For this review, take the finished solid that the model builds, in its own axes (mm). A direction names the side the tool comes from. Coordinates: 2 decimals unless noted, no trailing zeros. Order: outer loops, then holes, each group sorted by start corner. A loop starts at its lowest first (then second) coordinate and runs counter-clockwise, first axis right, second up.
Autodesk Fusion 360 part; units mm, degrees
sketch "Sketch1" plane through (0, 0, 0) normal (0, 0, 1) x (1, 0, 0)
  line L0 (20, -20) -> (-20, -20)
  line L1 (-20, -20) -> (-20, 20)
  line L2 (-20, 20) -> (20, 20)
  line L3 (20, 20) -> (20, -20)
  line L4 (20, -20) -> (-20, 20) construction
  line L5 (-20, -20) -> (20, 20) construction
  line L6 (12.5, -12.5) -> (-12.5, -12.5) construction
  line L7 (-12.5, -12.5) -> (-12.5, 12.5) construction
  line L8 (-12.5, 12.5) -> (12.5, 12.5) construction
  line L9 (12.5, 12.5) -> (12.5, -12.5) construction
  line L10 (12.5, -12.5) -> (-12.5, 12.5) construction
  line L11 (-12.5, -12.5) -> (12.5, 12.5) construction
  circle A0 centre (-12.5, 12.5) radius 2.25
  circle A1 centre (12.5, 12.5) radius 2.25
  circle A2 centre (12.5, -12.5) radius 2.25
  circle A3 centre (-12.5, -12.5) radius 2.25
  dimension "d1" = 40
  dimension "d2" = 40
  dimension "d3" = 25
  dimension "d4" = 25
  dimension "d5" = 4.5
  dimension "d6" = 4.5
  dimension "d7" = 4.5
  dimension "d8" = 4.5
extrude "Extrude1" add sketch "Sketch1" along normal blind 4
sketch "Sketch2" plane through (0, 0, 4) normal (0, 0, 1) x (-1, 0, 0)
  circle A0 centre (12.5, 12.5) radius 2.25
  circle A1 centre (12.5, -12.5) radius 2.25
  circle A2 centre (-12.5, -12.5) radius 2.25
  circle A3 centre (-12.5, 12.5) radius 2.25
  line L0 (-20, -20) -> (20, -20)
  line L1 (20, -20) -> (20, 20)
  line L2 (20, 20) -> (-20, 20)
  line L3 (-20, 20) -> (-20, -20)
  circle A4 centre (0, 0) radius 10.3
  circle A5 centre (0, 0) radius 12.3
  dimension "d11" = 20.6
  dimension "d12" = 2
extrude "Extrude2" add sketch "Sketch2" along normal blind 30 contours A5
sketch "Sketch3" plane through (0, 0, 0) normal (1, 0, 0) x (0, 1, 0)
  line L0 (12.3, 34) -> (-12.3, 34)
  line L1 (-12.3, 4) -> (12.3, 4)
  line L2 (-12.3, 34) -> (12.3, 4) construction
  circle A0 centre (0, 19) radius 2.1
  dimension "d15" = 4.2
extrude "Extrude3" cut sketch "Sketch3" along normal through all and the other way through all
fillet "Fillet1" radius 2 1 edges at (11.4676, -4.4479, 4)
1. Take a section at C-C, the plane x = 0. Give the boundary of the cut face in (y, z).
Answer below:
outline: (-20, 0) - (20, 0) - (20, 4) - (14.3, 4) arc R2 cw to (12.3, 6) - (12.3, 34) - (10.3, 34) - (10.3, 4) - (-10.3, 4) - (-10.3, 34) - (-12.3, 34) - (-12.3, 6) arc R2 cw to (-14.3, 4) - (-20, 4) - close
2. Clearance check with flat-ended pins moving along their axes: pin 1 Ø6 at (x, y) = (-12.5, 12.5) entering from -Z; pin 2 Ø6 at (x, y) = (-4, 3.5) entering from +Z; pin 3 Ø8 at (x, z) = (4, 10) entering from -Y; pin 4 Ø6.5 at (y, z) = (0, 19) entering from +X. State where each tip first meets the part, or that it passes through.
Answer below:
pin 1: stops at z = 0
pin 2: stops at z = 4
pin 3: stops at y = -12.3
pin 4: stops at x = 12.3
3. Take a section at B-B, the plane z = 13.5. Give the boundary of the cut face in (x, y), plus the area to 3 significant figures.
Answer below:
outline: circle Ø24.6 at (0, 0); hole circle Ø20.6 at (0, 0)
area: 142 mm2
4. To check wall thickness, follow L1, parallel to Y at x = 12.5, z = 0.8; L2, parallel to Z at x = 11.25, y = 0; L3, parallel to X at y = -12, z = 2. State the ranges of each line that lie inside material, in increasing order.
Answer below:
L1: y = -20 to -14.75, -10.25 to 10.25, 14.75 to 20
L2: z = 0 to 16.9, 21.1 to 34
L3: x = -20 to -14.69, -10.31 to 10.31, 14.69 to 20
5. Take a section at D-D, the plane x = -11.5. Give the number of separate pieces and of enclosed holes in the cut face, plus the area to 3 significant figures.
Answer below:
separate pieces: 3
enclosed holes: 1
area: 380 mm2
6. The part is to be moulded in two halves that separate along Y. For faces 1 (the face through (-5.4, 9.1, 34)), 2 (the face through (0, -20, 2)), 3 (the face through (-14.16, -14.02, 1.97)), 4 (the face through (11.18, -2.1, 18.91)), say which applies: +Y half, -Y half, draft (parallel to the pull), parting line (faces both ways), or undercut.
Answer below:
face 1: draft
face 2: -Y half
face 3: undercut
face 4: undercut
7. Take a section at A-A, the plane y = 0. Give the boundary of the cut face in (x, z).
Answer below:
outline: (-20, 0) - (20, 0) - (20, 4) - (14.3, 4) arc R2 cw to (12.3, 6) - (12.3, 16.9) - (10.3, 16.9) - (10.3, 4) - (-10.3, 4) - (-10.3, 16.9) - (-12.3, 16.9) - (-12.3, 6) arc R2 cw to (-14.3, 4) - (-20, 4) - close; (-12.3, 21.1) - (-10.3, 21.1) - (-10.3, 34) - (-12.3, 34) - close; (10.3, 21.1) - (12.3, 21.1) - (12.3, 34) - (10.3, 34) - close
8. Machinability: for faces 5 (the face through (0, 0, 4)), 6 (the face through (-14.16, 10.98, 1.97)), which of the approach directions +Z, -Z, +X, -X, +Y, -Y give a long, thin tool a straight path to every point of the face, cutting with its end or side? Answer none if there is none.
Answer below:
face 5: +Z
face 6: +Z, -Z
